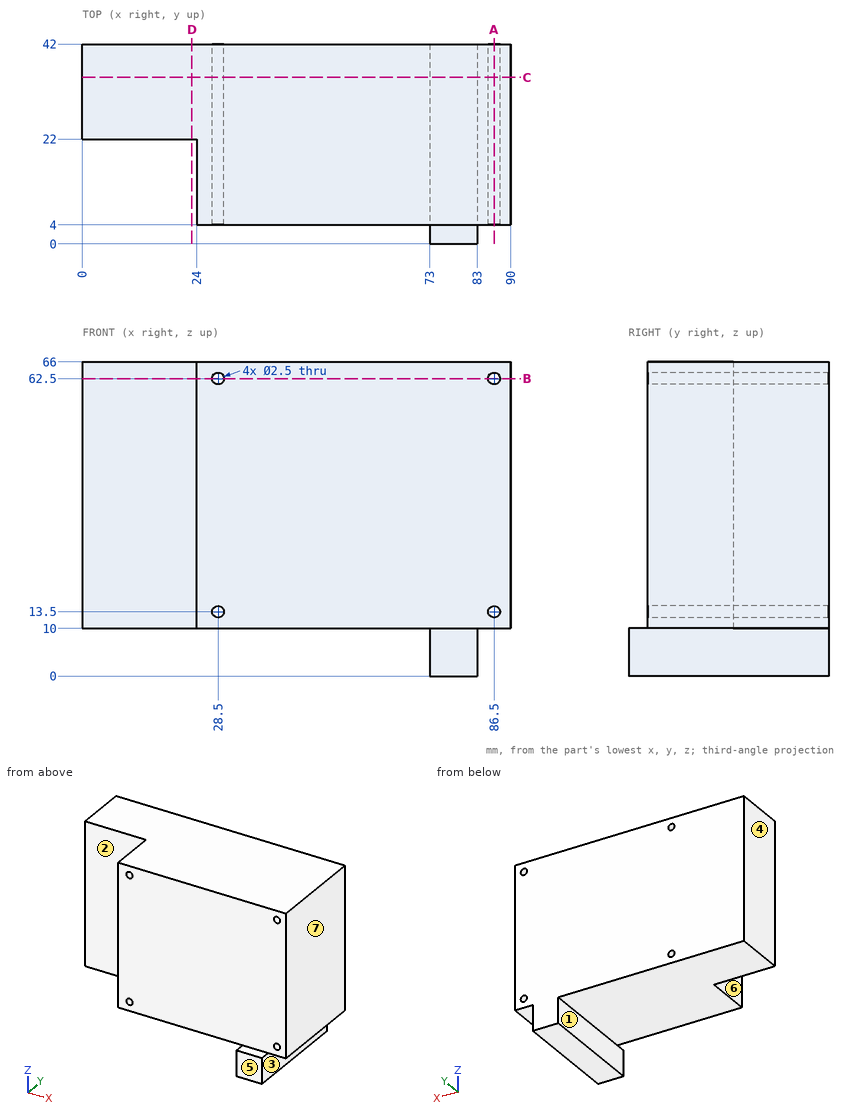
Part print with two shaded views. Sizes in mm from the minimum x, y, z corner. A direction names the side the tool comes from. Coordinates: 2 decimals unless noted, no trailing zeros. Write each loop counter-clockwise with the first axis right and the second up, starting at its lowest first coordinate (ties: lowest second). Pieces come first, ordered by that corner, then holes. Notation, with made-up numbers: (9, 89.5) - (65, 89.5) arc R16 ccw to (65, 95.5) - close; hole circle Ø2 at (54, -12.75). An arc over 180 degrees is marked (long way). Use a Markdown table: item, result. Add a question column.
Item 1: Drill centre lines: line 1 along Z through (x, y) = (86.5, 30); line 2 along X through (y, z) = (29, 62.5); line 3 along X through (y, z) = (20.5, 62.5). Where is each one in solid material? Low to high.
Item 2: Band-saw the part on B-B, the plane z = 62.5. Write the cut outline in (x, y).
Item 3: Two-plate mould, pull along X, no slides. Class the marked faces 5, 6 and 7: pulls with the +X half, pulls with the -X half, needs draft (parallel to the pull), parting line crosses it, or undercut.
Item 4: Band-saw the part on C-C, the plane y = 35. Write the cut outline in (x, z).
Item 5: Band-saw the part on D-D, the plane x = 23. Write the cut outline in (y, z), and give its area (3 significant figures).
Item 6: Band-saw the part on A-A, the plane x = 86.5. Write the cut outline in (y, z), and give its area (3 significant figures).
Item 7: Drop flat-ended pins along their axis: pin 1 (14.5 mm diameter, centred on y = 10.5, z = 25, fed in from -X); pin 2 (5 mm diameter, centred on y = 21, z = 6, fed in from -X); pin 3 (6 mm diameter, centred on x = 77.5, z = 55.5, fed in from -Y); pin 4 (4 mm diameter, centred on x = 28.5, z = 62.5, fed in from +Y). Give the stop position or say it passes through.
Item 8: 3-axis set-ups, long thin cutter, end or side, ignore diameter. For the marked faces 1, 2, 3 and 4: which of +Z, -Z, +X, -X, +Y, -Y reach the whole face in a straight line?
A:
| question | item | result |
|---|---|---|
| 1 | line 1 | z = 10 to 12.25, 14.75 to 61.25, 63.75 to 66 |
| 1 | line 2 | x = 0 to 27.25, 29.75 to 85.25, 87.75 to 90 |
| 1 | line 3 | x = 24 to 27.25, 29.75 to 85.25, 87.75 to 90 |
| 2 | outline | (0, 22) - (24, 22) - (24, 4) - (27.25, 4) - (27.25, 42) - (0, 42) - close; (29.75, 4) - (85.25, 4) - (85.25, 42) - (29.75, 42) - close; (87.75, 4) - (90, 4) - (90, 42) - (87.75, 42) - close |
| 3 | face 5 | needs draft |
| 3 | face 6 | pulls with the -X half |
| 3 | face 7 | pulls with the +X half |
| 4 | outline | (0, 10) - (73, 10) - (73, 0) - (83, 0) - (83, 10) - (90, 10) - (90, 66) - (0, 66) - close; hole circle Ø2.5 at (28.5, 13.5); hole circle Ø2.5 at (28.5, 62.5); hole circle Ø2.5 at (86.5, 13.5); hole circle Ø2.5 at (86.5, 62.5) |
| 5 | outline | (22, 10) - (42, 10) - (42, 66) - (22, 66) - close |
| 5 | area | 1,120 mm² |
| 6 | outline | (4, 10) - (42, 10) - (42, 12.25) - (4, 12.25) - close; (4, 14.75) - (42, 14.75) - (42, 61.25) - (4, 61.25) - close; (4, 63.75) - (42, 63.75) - (42, 66) - (4, 66) - close |
| 6 | area | 1,940 mm² |
| 7 | pin 1 | stops at x = 24 |
| 7 | pin 2 | stops at x = 73 |
| 7 | pin 3 | stops at y = 4 |
| 7 | pin 4 | stops at y = 42 |
| 8 | face 1 | -Z, -X, +Y, -Y |
| 8 | face 2 | +Z, -Z, -X, -Y |
| 8 | face 3 | -Z, +X, +Y, -Y |
| 8 | face 4 | +Z, -Z, -X, +Y, -Y |
